from build123d import *

# Parameters (mm, degrees)
SKETCH2_R = 1.25


with BuildPart() as part:
    # Sweep1: sweep along a path in Sketch1
    with BuildLine(Plane(origin=(0, 0, 0), x_dir=(1, 0, 0), z_dir=(0, 1, 0))) as sweep1_path:
        Line((-8, 0), (-4.649084765, 0))
        ThreePointArc((-4.649084765, 0), (-1.616920267, -1.391172972), (-0.693888418, -4.597010769))
        Line((-0.693888418, -4.597010769), (-7.486341248, -49.597010769))
        ThreePointArc((-7.486341248, -49.597010769), (-8.832710567, -52.032164497), (-11.441537595, -53))
        Line((-11.441537595, -53), (-17, -53))
    # Sketch2 → Sweep1 (sweep)
    with BuildSketch(Plane.ZY.offset(8)):
        Circle(SKETCH2_R)
    sweep(path=sweep1_path.line)


solid = part.part
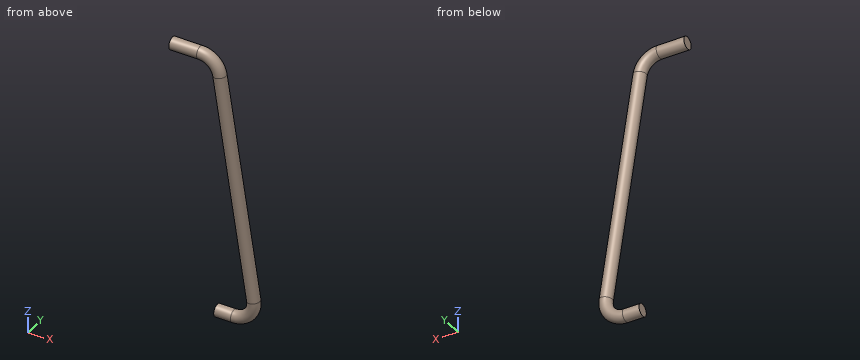
Model file for the job. Use its own axes, mm. Give positions to 0.01 mm unless a question says otherwise; leave off trailing zeros. Write each loop counter-clockwise with the first axis right and the second up, starting at its lowest first coordinate (ties: lowest second). Pieces come first, ordered by that corner, then holes. Notation, with made-up numbers: (86.5, -13.75) - (123.5, -13.75) arc R13 ccw to (123.5, -0.75) - close; hole circle Ø2 at (-40, 65). An arc over 180 degrees is marked (long way). Answer as CSV lines item,"result".
1. Band-saw the part on A-A (y = 0). Write the cut outline in (x, z), and give its area (3 significant figures).
Responses:
outline,"(-17, 51.75) - (-11.44, 51.75) arc R2.75 cw to (-8.72, 49.41) - (-1.93, 4.41) arc R2.75 cw to (-4.65, 1.25) - (-8, 1.25) - (-8, -1.25) - (-4.65, -1.25) arc R5.25 ccw to (0.54, 4.78) - (-6.25, 49.78) arc R5.25 ccw to (-11.44, 54.25) - (-17, 54.25) - close"
area,"167 mm2"
2. Pin check, flat tips, straight feed: pin 1 (6 mm diameter, centred on x = -2.5, z = 40.5, fed in from +Y); pin 2 (0.8 mm diameter, centred on y = -0.5, z = -0.5, fed in from -X). Stop position of each tip, or through.
Responses:
pin 1,"stops at y = 1.11"
pin 2,"stops at x = -8"
3. Drill centre lines: L1, parallel to X at y = 0.1, z = 31; L2, parallel to Z at x = -15.25, y = 0.75; L3, parallel to Z at x = -15.75, y = 0.2. Where is each one in solid material? Low to high. Write a range as [from, to].
Responses:
L1,"x = [-5.94, -3.42]"
L2,"z = [52, 54]"
L3,"z = [51.77, 54.23]"
